Autodesk Fusion 360 part; units mm, degrees
sketch "Эскиз1" plane through (0, 0, 0) normal (0, 1, 0) x (1, 0, 0)
  line L0 (36.85, -15.05) -> (-36.85, -15.05)
  line L1 (-36.85, -15.05) -> (-36.85, 15.05)
  line L2 (-36.85, 15.05) -> (36.85, 15.05)
  line L3 (36.85, 15.05) -> (36.85, -15.05)
  line L4 (36.85, -15.05) -> (-36.85, 15.05) construction
  line L5 (-36.85, -15.05) -> (36.85, 15.05) construction
  circle A0 centre (0.65, 4.55) radius 1.5
  dimension "d1" = 73.7
  dimension "d2" = 30.1
  dimension "d3" = 3
  dimension "d4" = 37.5
  dimension "d5" = 10.5
extrude "Выдавливание2" add sketch "Эскиз1" along normal blind 1.6
sketch "Эскиз2" plane through (0, 1.6, 0) normal (0, 1, 0) x (-1, 0, 0)
  line L0 (34.65, 4.05) -> (28.45, 4.05)
  line L1 (28.45, 4.05) -> (28.45, 10.25)
  line L2 (28.45, 10.25) -> (34.65, 10.25)
  line L3 (34.65, 10.25) -> (34.65, 4.05)
  circle A0 centre (-0.65, -4.55) radius 1.5
  circle A1 centre (-0.65, -4.55) radius 1.5
  line L4 (-36.85, -15.05) -> (36.85, -15.05)
  line L5 (36.85, -15.05) -> (36.85, 15.05)
  line L6 (36.85, 15.05) -> (-36.85, 15.05)
  line L7 (-36.85, 15.05) -> (-36.85, -15.05)
  line L8 (19.95, 4.05) -> (13.75, 4.05)
  line L9 (19.95, 10.25) -> (19.95, 4.05)
  line L10 (13.75, 10.25) -> (19.95, 10.25)
  line L11 (13.75, 4.05) -> (13.75, 10.25)
  line L12 (5.15, 4.05) -> (-1.05, 4.05)
  line L13 (5.15, 10.25) -> (5.15, 4.05)
  line L14 (-1.05, 10.25) -> (5.15, 10.25)
  line L15 (-1.05, 4.05) -> (-1.05, 10.25)
  line L16 (-9.85, 4.05) -> (-16.05, 4.05)
  line L17 (-9.85, 10.25) -> (-9.85, 4.05)
  line L18 (-16.05, 4.05) -> (-16.05, 10.25)
  line L19 (-16.05, 10.25) -> (-9.85, 10.25)
  line L20 (-24.65, 4.05) -> (-30.85, 4.05)
  line L21 (-24.65, 10.25) -> (-24.65, 4.05)
  line L22 (-30.85, 4.05) -> (-30.85, 10.25)
  line L23 (-30.85, 10.25) -> (-24.65, 10.25)
  dimension "d8" = 6.2
  dimension "d9" = 6.2
  dimension "d18" = 2.2
  dimension "d19" = 4.8
  dimension "d20" = 6.2
  dimension "d21" = 6.2
  dimension "d22" = 8.5
  dimension "d23" = 6.2
  dimension "d24" = 6.2
  dimension "d25" = 8.6
  dimension "d26" = 6.2
  dimension "d27" = 6.2
  dimension "d28" = 6.2
  dimension "d29" = 6.2
  dimension "d30" = 8.6
  dimension "d31" = 8.8
  dimension "d32" = 65.5
  dimension "d33" = 21
  dimension "d34" = 21.2
  dimension "d35" = 21
  dimension "d36" = 20.9
  dimension "d37" = 6
extrude "Выдавливание3" add sketch "Эскиз2" along normal blind 3.6 contours L0 L1 L2 L3 | L8 L9 L10 L11 | L12 L13 L14 L15 | L16 L17 L18 L19 | L20 L21 L22 L23
sketch "Эскиз3" plane through (0, 5.2, 0) normal (0, 1, 0) x (-1, 0, 0)
  line L0 (34.65, 10.25) -> (28.45, 10.25)
  line L1 (28.45, 10.25) -> (28.45, 4.05)
  line L2 (28.45, 4.05) -> (34.65, 4.05)
  line L3 (34.65, 4.05) -> (34.65, 10.25)
  line L4 (13.75, 4.05) -> (19.95, 4.05)
  line L5 (19.95, 4.05) -> (19.95, 10.25)
  line L6 (19.95, 10.25) -> (13.75, 10.25)
  line L7 (13.75, 10.25) -> (13.75, 4.05)
  line L8 (-1.05, 4.05) -> (5.15, 4.05)
  line L9 (5.15, 4.05) -> (5.15, 10.25)
  line L10 (5.15, 10.25) -> (-1.05, 10.25)
  line L11 (-1.05, 10.25) -> (-1.05, 4.05)
  line L12 (-16.05, 10.25) -> (-16.05, 4.05)
  line L13 (-16.05, 4.05) -> (-9.85, 4.05)
  line L14 (-9.85, 4.05) -> (-9.85, 10.25)
  line L15 (-9.85, 10.25) -> (-16.05, 10.25)
  line L16 (-30.85, 10.25) -> (-30.85, 4.05)
  line L17 (-30.85, 4.05) -> (-24.65, 4.05)
  line L18 (-24.65, 4.05) -> (-24.65, 10.25)
  line L19 (-24.65, 10.25) -> (-30.85, 10.25)
  circle A0 centre (31.55, 7.15) radius 1.7
  circle A1 centre (16.85, 7.15) radius 1.7
  circle A2 centre (2.05, 7.15) radius 1.7
  circle A3 centre (-12.95, 7.15) radius 1.7
  circle A4 centre (-27.75, 7.15) radius 1.7
  dimension "d40" = 3.4
  dimension "d41" = 3.4
  dimension "d42" = 3.4
  dimension "d43" = 3.4
  dimension "d44" = 3.4
extrude "Выдавливание4" add sketch "Эскиз3" along normal blind 1.4 contours A0 | A1 | A2 | A3 | A4
Geometry: final body of the model. Coordinates: model frame, mm. A direction names the side the tool comes from. Coordinates: 2 decimals unless noted, no trailing zeros. Order: outer loops, then holes, each group sorted by start corner. A loop starts at its lowest first (then second) coordinate and runs counter-clockwise, first axis right, second up. Notation, with made-up numbers: M 13.25,24.5 L 22.25,24.5 A28 ccw 22.25,54.5 Z; hole C 79.5,14 d6. An arc over 180 degrees is marked long. Answer in a Markdown table with one row per item. Add a question column.
Q1. Section query D-D on z = 13.5. Return the cut outline in (x, y), and give its area (3 significant figures).
Q2. Section query B-B on z = -4.55. Return the cut outline in (x, y).
Q3. Reachability of faces 1 (the flat face through (-32, 3, 10.25)), 2 (the flat face through (16.05, 3, 7)), 3 (the flat face through (-0.6, 5.2, 5.8)), 4 (the flat face through (-2, 3, 4.05)) from +Z, -Z, +X, -X, +Y, -Y: full face, straight path, thin tool, end or side. Return the list, or none.
Q4. Contact query for flat-ended pins moving along their axis: P1, Ø1.1, axis at x = -32, y = 4, coming from the +Z side; P2, Ø1.1, axis at y = 3, z = 8, coming from the -X side; P3, Ø1.1, axis at y = 3, z = 5.5, coming from the +X side. Output: stop coordinate, or through.
Q5. Line query: L1, parallel to X at y = 4.5, z = 10; L2, parallel to X at y = 0.9, z = -4.55; L3, parallel to Z at x = 0.65, y = 0.55. Output: solid intervals per line, ascending.
Q6. Section query A-A on y = 4.25. Return the cut outline in (x, z), and give its area (3 significant figures).
Q7. Section query C-C on x = -3. Return the cut outline in (y, z).
Completed:
| question | item | result |
|---|---|---|
| 1 | outline | M -36.85,0 L 36.85,0 L 36.85,1.6 L -36.85,1.6 Z |
| 1 | area | 118 mm2 |
| 2 | outline | M -36.85,0 L -0.85,0 L -0.85,1.6 L -36.85,1.6 Z; M 2.15,0 L 36.85,0 L 36.85,1.6 L 2.15,1.6 Z |
| 3 | face 1 | +Z, +X, -X, +Y |
| 3 | face 2 | +Z, -Z, +Y |
| 3 | face 3 | +Y |
| 3 | face 4 | -Z, +X, -X, +Y |
| 4 | P1 | stops at z = 10.25 |
| 4 | P2 | stops at x = -34.65 |
| 4 | P3 | stops at x = 30.85 |
| 5 | L1 | x = -34.65 to -28.45, -19.95 to -13.75, -5.15 to 1.05, 9.85 to 16.05, 24.65 to 30.85 |
| 5 | L2 | x = -36.85 to -0.85, 2.15 to 36.85 |
| 5 | L3 | z = -15.05 to -6.05, -3.05 to 15.05 |
| 6 | outline | M -34.65,4.05 L -28.45,4.05 L -28.45,10.25 L -34.65,10.25 Z; M -19.95,4.05 L -13.75,4.05 L -13.75,10.25 L -19.95,10.25 Z; M -5.15,4.05 L 1.05,4.05 L 1.05,10.25 L -5.15,10.25 Z; M 9.85,4.05 L 16.05,4.05 L 16.05,10.25 L 9.85,10.25 Z; M 24.65,4.05 L 30.85,4.05 L 30.85,10.25 L 24.65,10.25 Z |
| 6 | area | 192 mm2 |
| 7 | outline | M 0,-15.05 L 1.6,-15.05 L 1.6,4.05 L 5.2,4.05 L 5.2,5.74 L 6.6,5.74 L 6.6,8.56 L 5.2,8.56 L 5.2,10.25 L 1.6,10.25 L 1.6,15.05 L 0,15.05 Z |
